```python
from build123d import *

# Parameters (mm, degrees)
F0_W          = 200
F0_H          = 40
F1_DEPTH      = 10
F2_R          = 15
F3_DEPTH      = 10
F5_DEPTH      = 25
F6_R          = 15
F6_R_2        = 12
F7_DEPTH      = 5
F7_DEPTH_BACK = 5
F8_R          = 10
F9_R          = 2


with BuildPart() as f1:
    # F0 (on Top) → F1 (new body)
    with BuildSketch(Plane.XY):
        Rectangle(F0_W, F0_H)
    extrude(amount=F1_DEPTH)

    # F2 (on face) → F3 (cut)
    with BuildSketch(Plane.XY.offset(10)):
        with Locations((80, 0)):
            Circle(F2_R)
        with Locations((-80, 0)):
            Circle(F2_R)
    extrude(amount=-F3_DEPTH, mode=Mode.SUBTRACT)

    # F4 (on face) → F5 (cut)
    with BuildSketch(Plane.XY.offset(10)):
        with BuildLine():
            Line((-65.8578643763, -5), (65.8578643763, -5))
            ThreePointArc((65.8578643763, -5), (65, 0), (65.8578643763, 5))
            Line((65.8578643763, 5), (-65.8578643763, 5))
            ThreePointArc((-65.8578643763, 5), (-65.2160216052, 2.5365296809), (-65, 0))
            ThreePointArc((-65, 0), (-65.2160216052, -2.5365296809), (-65.8578643763, -5))
        make_face()
    extrude(amount=-F5_DEPTH, mode=Mode.SUBTRACT)

    # F6 (on face) → F7 (join, two sides)
    with BuildSketch(Plane.XY.offset(10)) as f7_sk:
        with Locations((-80, 0)):
            Circle(F6_R)
        with Locations((-80, 0)):
            Circle(F6_R_2, mode=Mode.SUBTRACT)
        with Locations((80, 0)):
            Circle(F6_R)
        with Locations((80, 0)):
            Circle(F6_R_2, mode=Mode.SUBTRACT)
    extrude(amount=F7_DEPTH)
    extrude(f7_sk.sketch, amount=-F7_DEPTH_BACK)

    # F8
    f8_edges = [f1.edges().sort_by_distance(p)[0] for p in [
        (-100, -20, 5),
        (100, -20, 5),
        (100, 20, 5),
        (-100, 20, 5),
    ]]
    fillet(f8_edges, radius=F8_R)

    # F9
    f9_edges = [f1.edges().sort_by_distance(p)[0] for p in [
        (0, -5, 0),
        (0, 5, 0),
    ]]
    fillet(f9_edges, radius=F9_R)


solid = f1.part
```
Read the model definition and answer for the solid it produces. Units are mm, in the model's axes. A direction names the side the tool comes from. Give positions to 0.01 mm unless a question says otherwise; leave off trailing zeros. Write each loop counter-clockwise with the first axis right and the second up, starting at its lowest first coordinate (ties: lowest second). Pieces come first, ordered by that corner, then holes. Notation, with made-up numbers: M 44,-39 L 52,-39 A13 ccw 52,-33 Z; hole C -15,-40 d7. An arc over 180 degrees is marked long. Put each result on its own line as item: value. Start each with the question number.
1. The part is cut by section B-B, the plane z = 12.5. Give the vertices of the cut face in (x, y).
2. Which of the six approach directions +Z, -Z, +X, -X, +Y, -Y give full straight-line access (tool end or side, diameter ignored) to faces 1 (the flat face through (1, 5, 6)), 2 (the flat face through (-87, 10, 5)), 3 (the flat face through (-1, 9, 10)), 4 (the flat face through (-100, 0, 5))?
3. The part is cut by section A-A, the plane x = -80. Give the vertices of the cut face in (y, z), and give its area (3 significant figures).
4. The part is cut by section D-D, the plane x = 79.5. Give the vertices of the cut face in (y, z).
5. The part is cut by section C-C, the plane y = 2.5. Give the vertices of the cut face in (x, z), and give its area (3 significant figures).
6. Each of these flat-tipped pins is pushed along its axis until it touches: pin 1 Ø14.5 at (x, y) = (-80, 0) entering from -Z; pin 2 Ø3 at (y, z) = (15.5, 10.5) entering from +X; pin 3 Ø12 at (x, y) = (-49.5, -5.5) entering from +Z. Where does it stop, or does it pass through?
7. Consider line 1 along X through (y, z) = (0, 3.1); line 2 along Y through (x, z) = (80, 11.8); line 3 along X through (y, z) = (5.5, 13.5). Determine where each line is inside the solid, lowest interval first.
Final values:
1. outline: C -80,0 d30; C 80,0 d30; hole C -80,0 d24; hole C 80,0 d24
2. face 1: +Z, -Z
2. face 2: -Z
2. face 3: +Z
2. face 4: +Z, -Z, -X, +Y, -Y
3. outline: M -20,0 L -15,0 L -15,5 L -12,5 L -12,15 L -15,15 L -15,10 L -20,10 Z; M 12,5 L 15,5 L 15,0 L 20,0 L 20,10 L 15,10 L 15,15 L 12,15 Z
3. area: 160 mm²
4. outline: M -20,0 L -14.99,0 L -14.99,5 L -11.99,5 L -11.99,15 L -14.99,15 L -14.99,10 L -20,10 Z; M 11.99,5 L 14.99,5 L 14.99,0 L 20,0 L 20,10 L 14.99,10 L 14.99,15 L 11.99,15 Z
5. outline: M -100,0 L -94.79,0 L -94.79,5 L -91.74,5 L -91.74,15 L -94.79,15 L -94.79,10 L -100,10 Z; M -68.26,5 L -65.21,5 L -65.21,15 L -68.26,15 Z; M 65.21,5 L 68.26,5 L 68.26,15 L 65.21,15 Z; M 91.74,5 L 94.79,5 L 94.79,0 L 100,0 L 100,10 L 94.79,10 L 94.79,15 L 91.74,15 Z
5. area: 226 mm²
6. pin 1: passes through
6. pin 2: stops at x = 99.13
6. pin 3: stops at z = 10
7. line 1: x = -100 to -95, 95 to 100
7. line 2: y = -15 to -12, 12 to 15
7. line 3: x = -93.96 to -90.67, -69.33 to -66.04, 66.04 to 69.33, 90.67 to 93.96
